Autodesk Inventor part; units mm, degrees
ref_plane "YZ Plane" through (0, 0, 0) normal (1, 0, 0) x (0, 1, 0)
ref_plane "XZ Plane" through (0, 0, 0) normal (0, 1, 0) x (-1, 0, 0)
ref_plane "XY Plane" through (0, 0, 0) normal (0, 0, 1) x (1, 0, 0)
sketch "草圖1" plane through (0, 0, 0) normal (0, 0, 1) x (1, 0, 0)
  line L0 (0, 0) -> (-100, 0) construction
  line L1 (0, 25) -> (-100, 25)
  line L2 (-100, -25) -> (0, -25)
  arc A0 (0, -25) -> (0, 25) centre (0, 0) ccw
  arc A1 (-100, 25) -> (-100, -25) centre (-100, 0) ccw
  circle A2 centre (0, 0) radius 25
  line L3 (-25, 25) -> (-25, -25)
  point P0 (-50, 0)
  point P1 (25, 0)
  point P2 (-125, 0)
  dimension "d0" = 50
  dimension "d1" = 150
extrude "擠出1" add sketch "草圖1" along normal mid plane 3 contours L3 L2 A1 L1
sketch "草圖2" plane through (-25, -25, 1.5) normal (1, 0, 0) x (0, 0, -1)
  circle A0 centre (-19, 25) radius 22
  line L0 (3, 50) -> (3, 0) construction
  point P0 (1.5, 25)
  point P1 (3, 25)
  dimension "d4" = 44
extrude "擠出2" add sketch "草圖2" against normal blind 3
fillet "圓角1" radius 20 2 edges at (-26.5, 11.0905, 1.5) (-26.5, -11.0905, 1.5)
sketch "草圖3" plane through (0, 0, 1.5) normal (0, 0, 1) x (1, 0, 0)
  line L0 (-94.9774, -1.6071) -> (-72.1571, -1.6071) construction
  line L1 (-72.1571, -1.6071) -> (-72.1571, -15.4278) construction
  line L2 (-72.1571, -15.4278) -> (-94.9774, -15.4278) construction
  line L3 (-94.9774, -15.4278) -> (-94.9774, -1.6071) construction
  point P0 (0, 0)
properties part number "Arm_4"
Work out the finished part from the listing and answer in its coordinate system (mm). A direction names the side the tool comes from. Round coordinates to 2 decimals unless told otherwise and drop trailing zeros. Loops run counter-clockwise (first coordinate to the right, second up) from the corner with the lowest first, then second, coordinate; pieces in that order, holes last. Notation, with made-up numbers: M -38,-38 L 3,-38 A15 cw 3,-19 Z; hole C -23,37 d6. An arc over 180 degrees is marked long. One line per question, with ' | ' between items.
Q1. The mould has two halves that part along Z. Classify faces 1 (the flat face through (-25, 0, 15)), 2 (the flat face through (-77, 0, 1.5)), 3 (the cylindrical face through (-26.521, 21.832, 8.602)): +Z half, -Z half, draft (parallel to the pull), parting line (faces both ways), or undercut.
Conclusion:
face 1: draft | face 2: +Z half | face 3: undercut
Q2. Find section C-C, the plane z = 20.5. Give the vertices of the cut face in (x, y).
Conclusion:
outline: M -28,-22 L -25,-22 L -25,22 L -28,22 Z
Q3. Each of these flat-tipped pins is pushed along its axis until it touches: pin 1 Ø5 at (x, y) = (-102, -19) entering from +Z; pin 2 Ø1.5 at (y, z) = (19, 16) entering from -X. Where does it stop, or does it pass through?
Conclusion:
pin 1: stops at z = 1.5 | pin 2: stops at x = -28
Q4. Consider line 1 along X through (y, z) = (-4.5, 19); line 2 along Z through (x, y) = (-69, 22). Determine where each line is inside the solid, lowest interval first. Write a range as from..to.
Conclusion:
line 1: x = -28..-25 | line 2: z = -1.5..1.5
Q5. Find section A-A, the plane x = -57. Give the vertices of the cut face in (y, z), then the cut area to 3 significant figures.
Conclusion:
outline: M -25,-1.5 L 25,-1.5 L 25,1.5 L -25,1.5 Z | area: 150 mm2
Q6. Find section B-B, the plane y = -19. Give the vertices of the cut face in (x, z), then the cut area to 3 significant figures.
Conclusion:
outline: M -116.25,-1.5 L -25,-1.5 L -25,31.59 L -28,31.59 L -28,1.5 L -116.25,1.5 Z | area: 364 mm2
Q7. A tool of negligible diameter and unlimited length cuts with its end or side. For faces 4 (the flat face through (-28, 0, 22)), 5 (the flat face through (-76, 0, -1.5)), from which of +Z, -Z, +X, -X, +Y, -Y can it reach the whole face along a straight path? Write none if from no direction.
Conclusion:
face 4: +Z, -X, +Y, -Y | face 5: -Z, +X, -X, +Y, -Y
Q8. Find section D-D, the plane y = -12.5. Give the vertices of the cut face in (x, z), then the cut area to 3 significant figures.
Conclusion:
outline: M -121.65,-1.5 L -25,-1.5 L -25,38.6 L -28,38.6 L -28,1.5 L -121.65,1.5 Z | area: 401 mm2
